Here's the drawing with two shaded views (mm, measured from the low corner). I have some questions. Give positions to 0.01 mm unless a question says otherwise; leave off trailing zeros. Write each loop counter-clockwise with the first axis right and the second up, starting at its lowest first coordinate (ties: lowest second). Pieces come first, ordered by that corner, then holes. Notation, with made-up numbers: (11, 46.25) -> (16, 46.25) arc R16 cw to (16, 69.25) -> close; hole circle Ø11 at (-12.5, -2.75). An arc over 180 degrees is marked (long way). One line per question, with ' | ' between items.
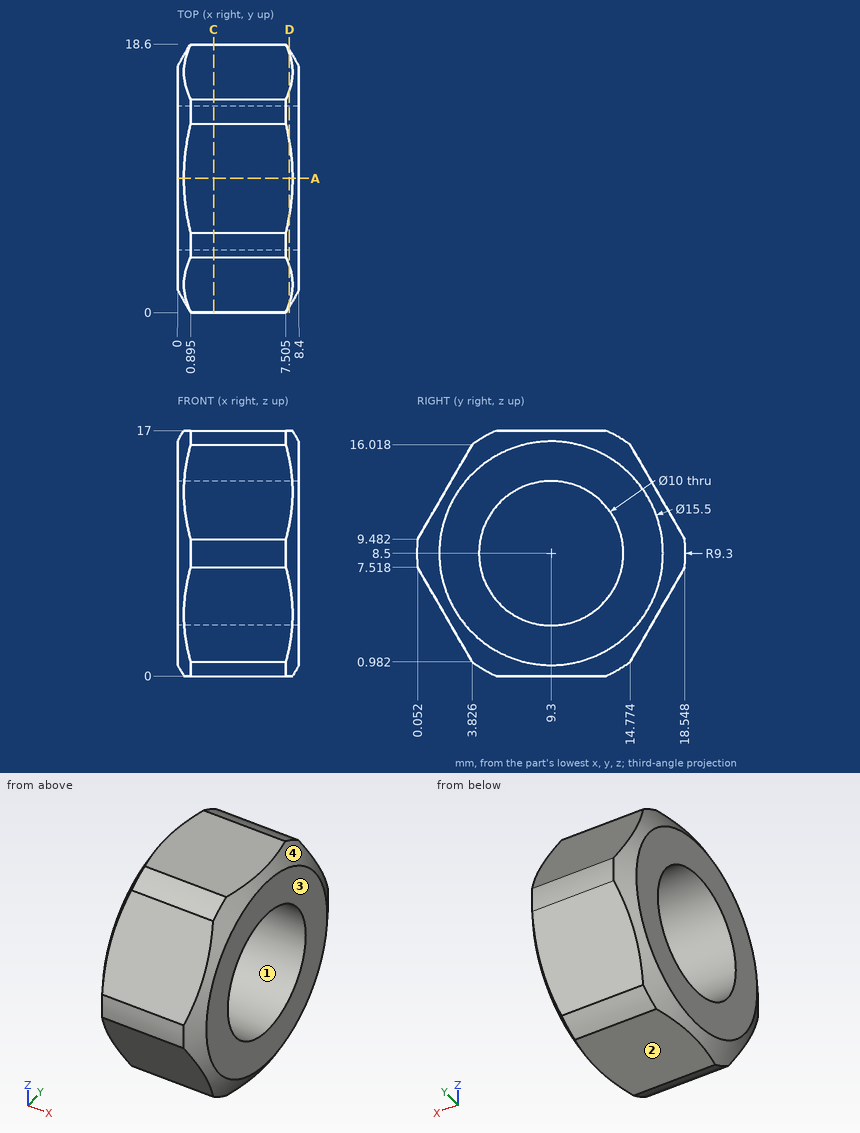
Q1. Will these pins go through, and if not, where does the flat tip stop? pin 1 (1 mm diameter, centred on x = 3.5, y = 14.5, fed in from -Z) (1 decimal); pin 2 (5 mm diameter, centred on x = 4, z = 3, fed in from -Y); pin 3 (1.5 mm diameter, centred on x = 4.5, z = 2, fed in from +Y) (1 decimal).
Answer below:
pin 1: stops at z = 0.5 | pin 2: stops at y = 1.22 | pin 3: stops at y = 15.8
Q2. Imagine slicing it at D-D on x = 7.75. Please give me the cut outline in (y, z) (1 decimal), and give its area (3 significant figures).
Answer below:
outline: (0.7, 6.5) -> (3.2, 2) arc R8.9 ccw to (6.7, 0) -> (11.9, 0) arc R8.9 ccw to (15.4, 2) -> (17.9, 6.5) arc R8.9 ccw to (17.9, 10.5) -> (15.4, 15) arc R8.9 ccw to (11.9, 17) -> (6.7, 17) arc R8.9 ccw to (3.2, 15) -> (0.7, 10.5) arc R8.9 ccw to start; hole circle Ø10 at (9.3, 8.5) | area: 161 mm^2
Q3. If we mould it in two halves opening along Z, with no side actions, what happens to the marked faces 1, 2, 3 and 4? For each: +Z half, -Z half, draft (parallel to the pull), parting line (faces both ways), or undercut.
Answer below:
face 1: undercut | face 2: -Z half | face 3: draft | face 4: parting line
Q4. Imagine slicing it at A-A on y = 9.3. Please give me the cut outline in (x, z).
Answer below:
outline: (0, 0.75) -> (0.43, 0) -> (7.97, 0) -> (8.4, 0.75) -> (8.4, 3.5) -> (0, 3.5) -> close; (0, 13.5) -> (8.4, 13.5) -> (8.4, 16.25) -> (7.97, 17) -> (0.43, 17) -> (0, 16.25) -> close
Q5. Imagine slicing it at C-C on x = 2.5. Please give me the cut outline in (y, z) (1 decimal), and give its area (3 significant figures).
Answer below:
outline: (0.1, 7.5) -> (3.8, 1) arc R9.3 ccw to (5.5, 0) -> (13.1, 0) arc R9.3 ccw to (14.8, 1) -> (18.5, 7.5) arc R9.3 ccw to (18.5, 9.5) -> (14.8, 16) arc R9.3 ccw to (13.1, 17) -> (5.5, 17) arc R9.3 ccw to (3.8, 16) -> (0.1, 9.5) arc R9.3 ccw to start; hole circle Ø10 at (9.3, 8.5) | area: 169 mm^2
Q6. If I drill on line 1 along Z through (x, y) = (5.5, 9.3); line 2 along Y through (x, z) = (8.25, 5.25); line 3 along Y through (x, z) = (7.75, 9.5), over which ranges is the centre line in solid material (lowest first)?
Answer below:
line 1: z = 0 to 3.5, 13.5 to 17 | line 2: y = 1.98 to 5.5, 13.1 to 16.62 | line 3: y = 0.48 to 4.4, 14.2 to 18.12
